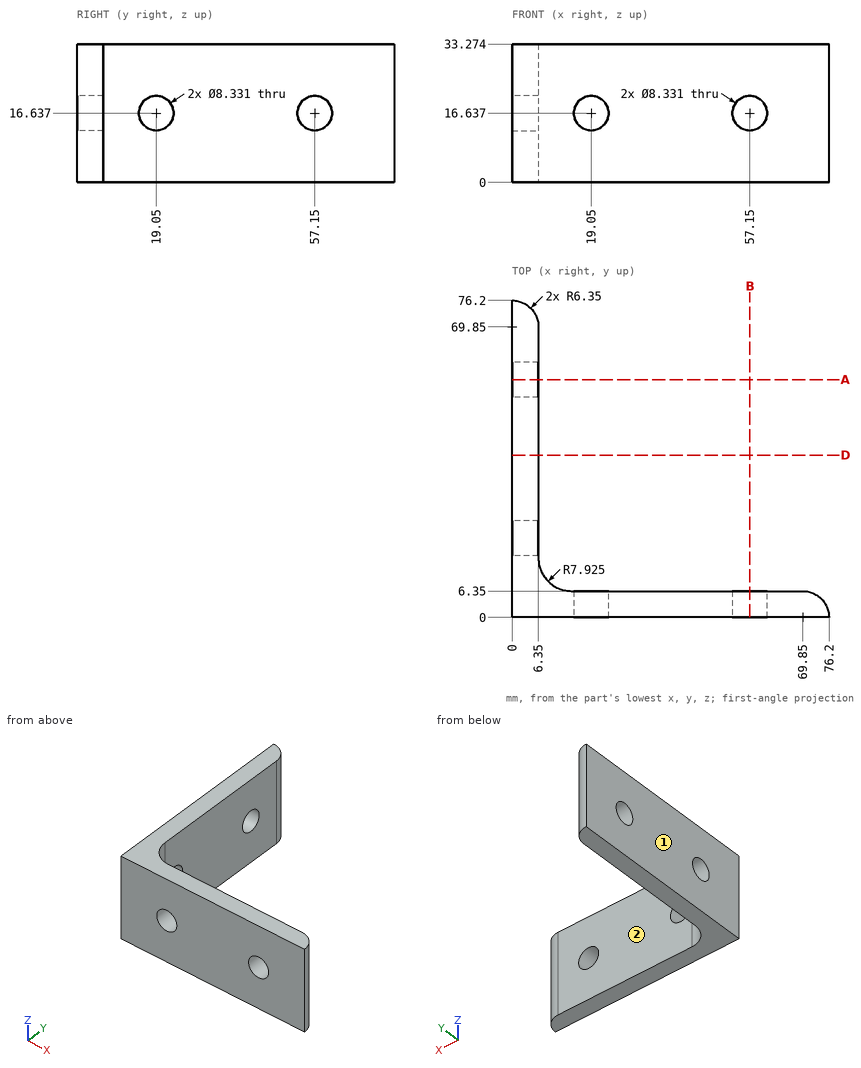
Geometry: see drawing. Coordinates: mm, zero at the bounding-box minimum. A direction names the side the tool comes from. Round coordinates to 2 decimals unless told otherwise and drop trailing zeros. Write each loop counter-clockwise with the first axis right and the second up, starting at its lowest first coordinate (ties: lowest second). Pieces come first, ordered by that corner, then holes.
Item 1: Section query D-D (y = 39). Return loops of the section in (x, z), plus the area to 3 significant figures.
Item 2: Section query A-A (y = 57.15). Return loops of the section in (x, z), plus the area to 3 significant figures.
Item 3: Material intervals for L1, parallel to Z at x = 19.05, y = 4.25; L2, parallel to Y at x = 60, z = 23.5, sorted ascending.
Item 4: Pin query (flat end, axial travel): P1, Ø10, axis at x = 34.5, z = 20, coming from the +Y side; P2, Ø3, axis at y = 63, z = 28, coming from the +X side. Return the tip coordinate at first contact, or that it passes through.
Item 5: Set-up query: the marked faces 1 and 2. Return all of +Z, -Z, +X, -X, +Y, -Y with unobstructed straight access to the full face (end or side cutting, diameter ignored); none if empty.
Completed:
1. outline: (0, 0) - (6.35, 0) - (6.35, 33.27) - (0, 33.27) - close
1. area: 211 mm2
2. outline: (0, 0) - (6.35, 0) - (6.35, 12.47) - (0, 12.47) - close; (0, 20.8) - (6.35, 20.8) - (6.35, 33.27) - (0, 33.27) - close
2. area: 158 mm2
3. L1: z = 0 to 12.47, 20.8 to 33.27
3. L2: y = 0 to 6.35
4. P1: stops at y = 6.35
4. P2: stops at x = 6.35
5. face 1: +Z, -Z, -X, +Y, -Y
5. face 2: +Z, -Z, +X, +Y
